Read the model definition and answer for the solid it produces. Units are mm, in the model's axes. Round coordinates to 2 decimals unless told otherwise and drop trailing zeros. Write each loop counter-clockwise with the first axis right and the second up, starting at its lowest first coordinate (ties: lowest second). Pieces come first, ordered by that corner, then holes.
Solid Edge part; units mm, degrees
sketch "Sketch1" plane through (0, 0, 0) normal (0, 0, 1) x (1, 0, 0)
  line L0 (0, 0) -> (100, 0)
  line L1 (100, 0) -> (100, 100)
  line L2 (100, 100) -> (0, 100)
  line L3 (0, 100) -> (0, 0)
  dimension "D1" = 100
extrude "Protrusion1" add sketch "Sketch1" along normal blind 5
sketch "Sketch2" plane through (50, 50, 5) normal (0, 0, 1) x (1, 0, 0)
  circle A0 centre (-30, 30) radius 4.6735
  circle A1 centre (30, 30) radius 4.6735
  circle A2 centre (30, -30) radius 4.6735
  circle A3 centre (-30, -30) radius 4.6735
extrude "Cutout1" cut sketch "Sketch2" against normal through all
fillet "Round_4" radius 5 4 edges at (100, 0, 2.5) (100, 100, 2.5) (0, 0, 2.5) (0, 100, 2.5)
Q1. Section B-B (z = 1.8) is taken. Determine the outline of the cut face in (x, y), then the cut area to 3 significant figures.
Verdict:
outline: (0, 5) arc R5 ccw to (5, 0) - (95, 0) arc R5 ccw to (100, 5) - (100, 95) arc R5 ccw to (95, 100) - (5, 100) arc R5 ccw to (0, 95) - close; hole circle Ø9.35 at (20, 20); hole circle Ø9.35 at (20, 80); hole circle Ø9.35 at (80, 20); hole circle Ø9.35 at (80, 80)
area: 9,700 mm2
Q2. Determine the mould class of faces 1 (the flat face through (49, 51, 0)), 2 (the cylindrical face through (24.317, 18.21, 2.535)), 3 (the cylindrical face through (98, 1, 3)) for opening direction X: pulls with the +X half, pulls with the -X half, needs draft (parallel to the pull), parting line crosses it, or undercut.
Verdict:
face 1: needs draft
face 2: undercut
face 3: pulls with the +X half
Q3. A flat-ended cylindrical pin translates along its axis: pin 1 Ø8.5 at (x, y) = (20, 80) entering from +Z. Find the tip coordinate at first contact, or state that the pin passes through.
Verdict:
pin 1: passes through
Q4. Straight lines are drawn through the part: probe 1 along Y at (x, z) = (20, 3.2); probe 2 along X at (y, z) = (22, 3.35); probe 3 along Y at (x, z) = (78.5, 2.55). For each, find the intervals that lie inside material, in ascending order.
Verdict:
probe 1: y = 0 to 15.33, 24.67 to 75.33, 84.67 to 100
probe 2: x = 0 to 15.78, 24.22 to 75.78, 84.22 to 100
probe 3: y = 0 to 15.57, 24.43 to 75.57, 84.43 to 100
Q5. Section A-A (x = 80) is taken. Determine the outline of the cut face in (y, z), then the cut area to 3 significant figures.
Verdict:
outline: (0, 0) - (15.33, 0) - (15.33, 5) - (0, 5) - close; (24.67, 0) - (75.33, 0) - (75.33, 5) - (24.67, 5) - close; (84.67, 0) - (100, 0) - (100, 5) - (84.67, 5) - close
area: 407 mm2
